Geometry: final body of the model. Coordinates: model frame, mm. Coordinates: 2 decimals unless noted, no trailing zeros. Write each loop counter-clockwise with the first axis right and the second up, starting at its lowest first coordinate (ties: lowest second). Pieces come first, ordered by that corner, then holes.
from build123d import *

# Parameters (mm, degrees)
SKETCH_R        = 2.75
SKETCH_R_2      = 8.1
PAD_DEPTH       = 10
SKETCH001_R     = 14
SKETCH001_R_2   = 8.1
PAD001_DEPTH    = 32
CHAMFER_SIZE    = 0.5
FILLET_R        = 0.5
CHAMFER001_SIZE = 0.5


with BuildPart() as part:
    # Sketch → Pad (new body)
    with BuildSketch(Plane.YZ):
        with BuildLine():
            ThreePointArc((-13.266499, 20), (-24, 0), (-13.266499, -20))
            Line((-13.266499, -20), (13.266499, -20))
            ThreePointArc((13.266499, -20), (24, 0), (13.266499, 20))
            Line((-13.266499, 20), (13.266499, 20))
        make_face()
        with Locations((-13.435058, 13.435)):
            Circle(SKETCH_R, mode=Mode.SUBTRACT)
        with Locations((-19, 0)):
            Circle(SKETCH_R, mode=Mode.SUBTRACT)
        with Locations((-13.435058, -13.435)):
            Circle(SKETCH_R, mode=Mode.SUBTRACT)
        with Locations((13.435058, 13.435)):
            Circle(SKETCH_R, mode=Mode.SUBTRACT)
        with Locations((19, 0)):
            Circle(SKETCH_R, mode=Mode.SUBTRACT)
        with Locations((13.435058, -13.435)):
            Circle(SKETCH_R, mode=Mode.SUBTRACT)
        Circle(SKETCH_R_2, mode=Mode.SUBTRACT)
    extrude(amount=PAD_DEPTH)

    # Sketch001 → Pad001 (new body)
    with BuildSketch(Plane.YZ.offset(10)):
        Circle(SKETCH001_R)
        Circle(SKETCH001_R_2, mode=Mode.SUBTRACT)
    extrude(amount=PAD001_DEPTH)

    # Chamfer
    chamfer_edges = [part.edges().sort_by_distance(p)[0] for p in [
        (0, -16.185058, -13.435),
        (10, -16.185058, -13.435),
        (0, -21.75, 0),
        (10, -21.75, 0),
        (0, -16.185058, 13.435),
        (10, -16.185058, 13.435),
        (0, 10.685058, 13.435),
        (10, 10.685058, 13.435),
        (0, 16.25, 0),
        (10, 16.25, 0),
        (0, 10.685058, -13.435),
        (10, 10.685058, -13.435),
    ]]
    chamfer(chamfer_edges, length=CHAMFER_SIZE)

    # Fillet
    fillet_edges = [part.edges().sort_by_distance(p)[0] for p in [
        (42, -14, 0),
    ]]
    fillet(fillet_edges, radius=FILLET_R)

    # Chamfer001
    chamfer001_edges = [part.edges().sort_by_distance(p)[0] for p in [
        (5, -13.266499, 20),
        (5, -13.266499, -20),
        (0, -24, 0),
        (10, -24, 0),
        (5, 13.266499, 20),
        (0, 0, 20),
        (10, 0, 20),
        (5, 13.266499, -20),
        (0, 24, 0),
        (10, 24, 0),
        (0, 0, -20),
        (10, 0, -20),
    ]]
    chamfer(chamfer001_edges, length=CHAMFER001_SIZE)


solid = part.part
Item 1: Pull-direction query (Y, two-part tool) for faces 1 (the cylindrical face through (25.53, 12.932, -5.362)), 2 (the flat face through (10, 4.9, 13.3)), 3 (the cylindrical face through (4.937, -21.747, 0.121)); classes: released by +Y, released by -Y, zero draft, split by the parting line, or undercut.
Derived:
face 1: split by the parting line
face 2: zero draft
face 3: undercut
Item 2: Section A-A, the plane y = 0. Output: boundary loops of the cut face in (x, z), plus the area to 3 significant figures.
Derived:
outline: (0, -19.5) - (0.5, -20) - (9.5, -20) - (10, -19.5) - (10, -14) - (41.5, -14) arc R0.5 ccw to (42, -13.5) - (42, -8.1) - (0, -8.1) - close; (0, 8.1) - (42, 8.1) - (42, 13.5) arc R0.5 ccw to (41.5, 14) - (10, 14) - (10, 19.5) - (9.5, 20) - (0.5, 20) - (0, 19.5) - close
area: 615 mm2
Item 3: Section B-B, the plane z = 0. State how many separate pieces and enclosed holes the cut face has, plus the area to 3 significant figures.
Derived:
separate pieces: 4
enclosed holes: 0
area: 584 mm2
Item 4: Section C-C, the plane x = 39.5. Output: boundary loops of the cut face in (y, z), plus the area to 3 significant figures.
Derived:
outline: circle Ø28 at (0, 0); hole circle Ø16.2 at (0, 0)
area: 410 mm2
Item 5: Pin query (flat end, axial travel): pin 1 (5 mm diameter, centred on y = 13.44, z = 13.44, fed in from -X); pin 2 (12 mm diameter, centred on x = 35, z = 3, fed in from +Y); pin 3 (2 mm diameter, centred on x = 19, y = 12, fed in from -Z); pin 4 (12 mm diameter, centred on x = 23, y = -17, fed in from +Z). Return the tip coordinate at first contact, or that it passes through.
Derived:
pin 1: passes through
pin 2: stops at y = 14
pin 3: stops at z = -8.66
pin 4: stops at z = 8.66
Item 6: Material intervals for probe 1 along Z at (x, y) = (11, 0); probe 2 along X at (y, z) = (-0.5, 17.5); probe 3 along Y at (x, z) = (7, 11.5), sorted ascending.
Derived:
probe 1: z = -14 to -8.1, 8.1 to 14
probe 2: x = 0 to 10
probe 3: y = -21.07 to -15.39, -11.48 to 11.48, 15.39 to 21.07
